Here's the drawing with two shaded views (mm, measured from the low corner). I have some questions. A direction names the side the tool comes from. Coordinates: 2 decimals unless noted, no trailing zeros. Write each loop counter-clockwise with the first axis right and the second up, starting at its lowest first coordinate (ties: lowest second). Pieces come first, ordered by that corner, then holes.
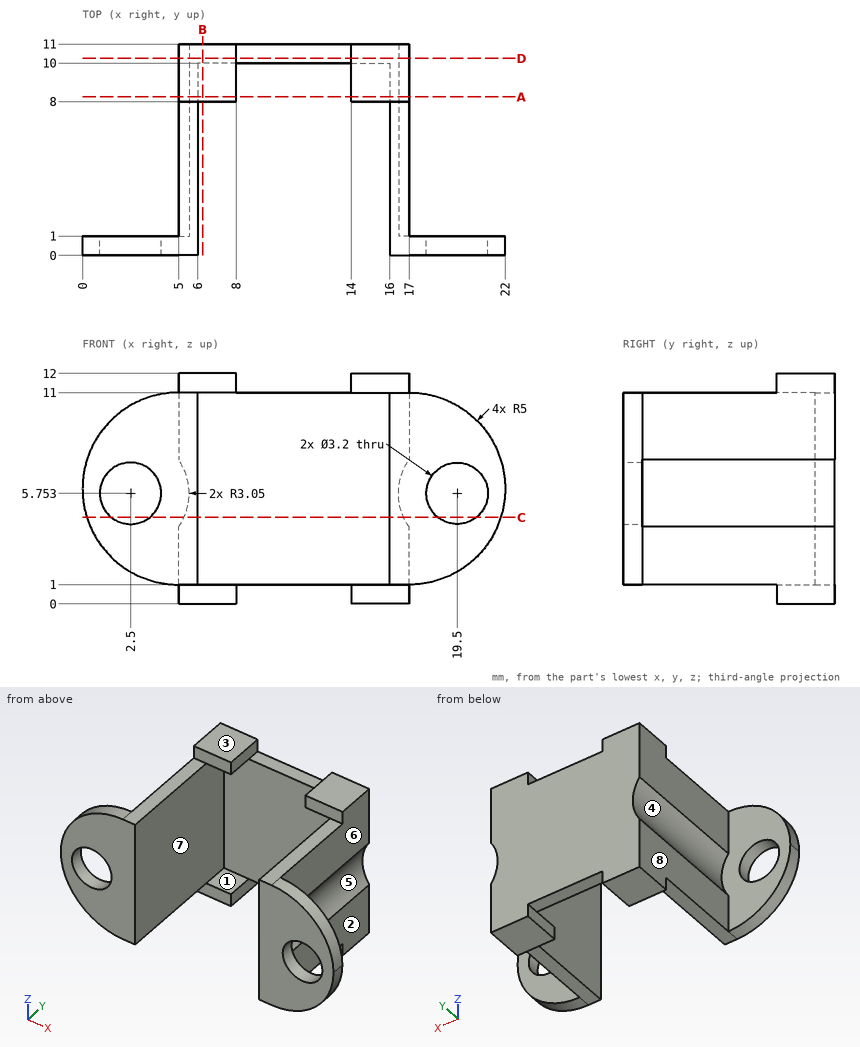
1. If we section it at B-B, the plane x = 6.25: List the corners of the cut face in (y, z) for me, plus the area to 3 significant figures.
2. I'm going to push flat-ended pins straight in: P1, Ø0.5, axis at x = 5.5, y = 5.5, coming from the -Z side; P2, Ø3.5, axis at y = 4, z = 11, coming from the -X side; P3, Ø0.5, axis at x = 5.5, y = 3, coming from the +Z side. Where does each tip first touch, or does it pass through?
3. Which directions (+Z, -Z, +X, -X, +Y, -Y) give clear straight access to the entire face, cutting with the end or side of a thin tool? Please do the marked faces 5, 6, 7 and 8.
4. If I drill on L1, parallel to X at y = 2, z = 8.5; L2, parallel to Y at x = 11.75, z = 7; L3, parallel to X at y = 8.25, z = 5.5, over which ranges is the centre line in solid material (lowest first)?
5. We'd pull the mould along Z, two halves only. Please class the marked faces 1, 2, 3 and 4: released by +Z, released by -Z, zero draft, split by the parting line, or undercut.
6. If we section it at C-C, the plane z = 4.5: List the corners of the cut face in (x, y) for me (1 decimal).
7. If we section it at D-D, the plane y = 10.25: List the corners of the cut face in (x, z) for me.
8. If we section it at A-A, the plane y = 8.25: List the corners of the cut face in (x, z) for me.
Answers:
1. outline: (8, 0) - (11, 0) - (11, 12) - (8, 12) - (8, 11) - (10, 11) - (10, 1) - (8, 1) - close
1. area: 16.0 mm2
2. P1: stops at z = 1
2. P2: stops at x = 5
2. P3: stops at z = 11
3. face 5: +X, +Y
3. face 6: +Z, -Z, +X, +Y
3. face 7: -Y
3. face 8: +Z, -Z, -X, +Y
4. L1: x = 5 to 6, 16 to 17
4. L2: y = 10 to 11
4. L3: x = 5.54 to 6, 16 to 16.46
5. face 1: undercut
5. face 2: zero draft
5. face 3: released by +Z
5. face 4: undercut
6. outline: (0.2, 0) - (1.5, 0) - (1.5, 1) - (0.2, 1) - close; (3.5, 0) - (6, 0) - (6, 10) - (16, 10) - (16, 0) - (18.5, 0) - (18.5, 1) - (16.7, 1) - (16.7, 11) - (5.3, 11) - (5.3, 1) - (3.5, 1) - close; (20.5, 0) - (21.8, 0) - (21.8, 1) - (20.5, 1) - close
7. outline: (5, 0) - (8, 0) - (8, 1) - (14, 1) - (14, 0) - (17, 0) - (17, 4.01) arc R3.05 cw to (17, 7.5) - (17, 12) - (14, 12) - (14, 11) - (8, 11) - (8, 12) - (5, 12) - (5, 7.5) arc R3.05 cw to (5, 4.01) - close
8. outline: (5, 0) - (8, 0) - (8, 1) - (6, 1) - (6, 11) - (8, 11) - (8, 12) - (5, 12) - (5, 7.5) arc R3.05 cw to (5, 4.01) - close; (14, 0) - (17, 0) - (17, 4.01) arc R3.05 cw to (17, 7.5) - (17, 12) - (14, 12) - (14, 11) - (16, 11) - (16, 1) - (14, 1) - close
